from build123d import *

# Parameters (mm, degrees)
SKETCH1_W           = 70.5
SKETCH1_H           = 60
SKETCH1_R           = 2.95
BOSS_EXTRUDE1_DEPTH = 10
SKETCH3_R           = 4.5
CUT_EXTRUDE1_DEPTH  = 5
SKETCH4_W           = 10
SKETCH4_H           = 60
BOSS_EXTRUDE3_DEPTH = 31
CUT_EXTRUDE2_REACH  = 103.248
SKETCH5_R           = 12.25
SKETCH5_R_2         = 2.25
SKETCH6_W           = 60
SKETCH6_H           = 31
SKETCH6_R           = 8
BOSS_EXTRUDE4_DEPTH = 5
SKETCH7_W           = 70.5
SKETCH7_H           = 60
BOSS_EXTRUDE5_DEPTH = 5
SKETCH8_W           = 60
SKETCH8_H           = 100
SKETCH8_R           = 2.25
SKETCH8_R_2         = 20.5
BOSS_EXTRUDE6_DEPTH = 10
CUT_EXTRUDE3_REACH  = 174.876
SKETCH10_W          = 50
SKETCH10_H          = 96
SKETCH10_R          = 2.5
BOSS_EXTRUDE7_DEPTH = 10
CHAMFER1_SIZE       = 50
SKETCH11_W          = 60.5
SKETCH11_H          = 50
BOSS_EXTRUDE8_DEPTH = 10
CUT_EXTRUDE4_REACH  = 194.552
SKETCH12_R          = 4.25
CUT_EXTRUDE6_REACH  = 190.59
SKETCH14_R          = 4.25


with BuildPart() as part:
    # Sketch1 → Boss-Extrude1 (new body)
    with BuildSketch(Plane(origin=(0, 0, 0), x_dir=(1, 0, 0), z_dir=(0, 1, 0))):
        with Locations((35.25, 30)):
            Rectangle(SKETCH1_W, SKETCH1_H)
        with Locations(Location((53.25, 46, 0), (0, 0, 270))):
            Circle(SKETCH1_R, mode=Mode.SUBTRACT)
        with Locations(Location((53.25, 14, 0), (0, 0, 270))):
            Circle(SKETCH1_R, mode=Mode.SUBTRACT)
        with Locations(Location((17.25, 46, 0), (0, 0, 270))):
            Circle(SKETCH1_R, mode=Mode.SUBTRACT)
        with Locations(Location((17.25, 14, 0), (0, 0, 270))):
            Circle(SKETCH1_R, mode=Mode.SUBTRACT)
    extrude(amount=BOSS_EXTRUDE1_DEPTH)

    # Sketch3 → Cut-Extrude1 (cut)
    with BuildSketch(Plane(origin=(0, 10, 0), x_dir=(1, 0, 0), z_dir=(0, 1, 0))):
        with Locations(Location((53.25, 46, 0), (0, 0, 270))):
            Circle(SKETCH3_R)
        with Locations(Location((53.25, 14, 0), (0, 0, 270))):
            Circle(SKETCH3_R)
        with Locations(Location((17.25, 46, 0), (0, 0, 270))):
            Circle(SKETCH3_R)
        with Locations(Location((17.25, 14, 0), (0, 0, 270))):
            Circle(SKETCH3_R)
    extrude(amount=-CUT_EXTRUDE1_DEPTH, mode=Mode.SUBTRACT)

    # Sketch4 → Boss-Extrude3 (add)
    with BuildSketch(Plane(origin=(0, 10, 0), x_dir=(1, 0, 0), z_dir=(0, 1, 0))):
        with Locations((5, 30)):
            Rectangle(SKETCH4_W, SKETCH4_H)
    extrude(amount=BOSS_EXTRUDE3_DEPTH)

    # Sketch5 → Cut-Extrude2 (cut, up to next)
    with BuildSketch(Plane.ZY, mode=Mode.PRIVATE) as cut_extrude2_sk1:
        with Locations((-30, 25)):
            Circle(SKETCH5_R)
    cut_extrude2_tool1 = extrude(cut_extrude2_sk1.sketch, amount=-CUT_EXTRUDE2_REACH, mode=Mode.PRIVATE) & part.part
    # Sketch5 → Cut-Extrude2 (cut, up to next)
    with BuildSketch(Plane.ZY, mode=Mode.PRIVATE) as cut_extrude2_sk2:
        with Locations((-14, 25)):
            Circle(SKETCH5_R_2)
    cut_extrude2_tool2 = extrude(cut_extrude2_sk2.sketch, amount=-CUT_EXTRUDE2_REACH, mode=Mode.PRIVATE) & part.part
    # Sketch5 → Cut-Extrude2 (cut, up to next)
    with BuildSketch(Plane.ZY, mode=Mode.PRIVATE) as cut_extrude2_sk3:
        with Locations((-18.686291501, 36.313708499)):
            Circle(SKETCH5_R_2)
    cut_extrude2_tool3 = extrude(cut_extrude2_sk3.sketch, amount=-CUT_EXTRUDE2_REACH, mode=Mode.PRIVATE) & part.part
    # Sketch5 → Cut-Extrude2 (cut, up to next)
    with BuildSketch(Plane.ZY, mode=Mode.PRIVATE) as cut_extrude2_sk4:
        with Locations((-18.686291501, 13.686291501)):
            Circle(SKETCH5_R_2)
    cut_extrude2_tool4 = extrude(cut_extrude2_sk4.sketch, amount=-CUT_EXTRUDE2_REACH, mode=Mode.PRIVATE) & part.part
    # Sketch5 → Cut-Extrude2 (cut, up to next)
    with BuildSketch(Plane.ZY, mode=Mode.PRIVATE) as cut_extrude2_sk5:
        with Locations((-41.313708499, 36.313708499)):
            Circle(SKETCH5_R_2)
    cut_extrude2_tool5 = extrude(cut_extrude2_sk5.sketch, amount=-CUT_EXTRUDE2_REACH, mode=Mode.PRIVATE) & part.part
    # Sketch5 → Cut-Extrude2 (cut, up to next)
    with BuildSketch(Plane.ZY, mode=Mode.PRIVATE) as cut_extrude2_sk6:
        with Locations((-46, 25)):
            Circle(SKETCH5_R_2)
    cut_extrude2_tool6 = extrude(cut_extrude2_sk6.sketch, amount=-CUT_EXTRUDE2_REACH, mode=Mode.PRIVATE) & part.part
    # Sketch5 → Cut-Extrude2 (cut, up to next)
    with BuildSketch(Plane.ZY, mode=Mode.PRIVATE) as cut_extrude2_sk7:
        with Locations((-41.313708499, 13.686291501)):
            Circle(SKETCH5_R_2)
    cut_extrude2_tool7 = extrude(cut_extrude2_sk7.sketch, amount=-CUT_EXTRUDE2_REACH, mode=Mode.PRIVATE) & part.part
    add(cut_extrude2_tool1.solids().sort_by_distance((0, 25, -30))[0], mode=Mode.SUBTRACT)
    add(cut_extrude2_tool2.solids().sort_by_distance((0, 25, -14))[0], mode=Mode.SUBTRACT)
    add(cut_extrude2_tool3.solids().sort_by_distance((0, 36.313708, -18.686292))[0], mode=Mode.SUBTRACT)
    add(cut_extrude2_tool4.solids().sort_by_distance((0, 13.686292, -18.686292))[0], mode=Mode.SUBTRACT)
    add(cut_extrude2_tool5.solids().sort_by_distance((0, 36.313708, -41.313708))[0], mode=Mode.SUBTRACT)
    add(cut_extrude2_tool6.solids().sort_by_distance((0, 25, -46))[0], mode=Mode.SUBTRACT)
    add(cut_extrude2_tool7.solids().sort_by_distance((0, 13.686292, -41.313708))[0], mode=Mode.SUBTRACT)

    # Sketch6 → Boss-Extrude4 (add)
    with BuildSketch(Plane(origin=(70.5, 0, 0), x_dir=(0, 0, -1), z_dir=(1, 0, 0))):
        with Locations((30, 25.5)):
            Rectangle(SKETCH6_W, SKETCH6_H)
        with Locations((30, 25)):
            Circle(SKETCH6_R, mode=Mode.SUBTRACT)
    extrude(amount=-BOSS_EXTRUDE4_DEPTH)

    # Sketch7 → Boss-Extrude5 (add)
    with BuildSketch(Plane(origin=(0, 41, 0), x_dir=(1, 0, 0), z_dir=(0, 1, 0))):
        with Locations((35.25, 30)):
            Rectangle(SKETCH7_W, SKETCH7_H)
    extrude(amount=BOSS_EXTRUDE5_DEPTH)

    # Sketch8 → Boss-Extrude6 (add)
    with BuildSketch(Plane.ZY):
        with Locations((-30, 96)):
            Rectangle(SKETCH8_W, SKETCH8_H)
        with Locations((-53.57, 72.43)):
            Circle(SKETCH8_R, mode=Mode.SUBTRACT)
        with Locations((-6.43, 72.43)):
            Circle(SKETCH8_R, mode=Mode.SUBTRACT)
        with Locations((-6.43, 119.57)):
            Circle(SKETCH8_R, mode=Mode.SUBTRACT)
        with Locations((-53.57, 119.57)):
            Circle(SKETCH8_R, mode=Mode.SUBTRACT)
        with Locations((-30, 96)):
            Circle(SKETCH8_R_2, mode=Mode.SUBTRACT)
    extrude(amount=-BOSS_EXTRUDE6_DEPTH)

    # Sketch9 → Cut-Extrude3 (cut, up to next)
    with BuildSketch(Plane.XY, mode=Mode.PRIVATE) as cut_extrude3_sk1:
        Polygon((10, 41), (65.5, 41), (65.5, 10), (70.5, 10), (70.5, 46), (10, 46), align=None)
    cut_extrude3_tool1 = extrude(cut_extrude3_sk1.sketch, amount=-CUT_EXTRUDE3_REACH, mode=Mode.PRIVATE) & part.part
    add(cut_extrude3_tool1.solids().sort_by_distance((37.75, 41.704006, 0))[0], mode=Mode.SUBTRACT)

    # Sketch10 → Boss-Extrude7 (add)
    with BuildSketch(Plane.ZY):
        with Locations((-85, 48)):
            Rectangle(SKETCH10_W, SKETCH10_H)
        with Locations((-65.555555556, 90.444444444)):
            Circle(SKETCH10_R, mode=Mode.SUBTRACT)
        with Locations((-104.444444444, 51.555555556)):
            Circle(SKETCH10_R, mode=Mode.SUBTRACT)
        with Locations((-98.888888889, 57.111111111)):
            Circle(SKETCH10_R, mode=Mode.SUBTRACT)
        with Locations((-93.333333333, 62.666666667)):
            Circle(SKETCH10_R, mode=Mode.SUBTRACT)
        with Locations((-87.777777778, 68.222222222)):
            Circle(SKETCH10_R, mode=Mode.SUBTRACT)
        with Locations((-87.777777778, 73.777777778)):
            Circle(SKETCH10_R, mode=Mode.SUBTRACT)
        with Locations((-98.888888889, 84.888888889)):
            Circle(SKETCH10_R, mode=Mode.SUBTRACT)
        with Locations((-104.444444444, 90.444444444)):
            Circle(SKETCH10_R, mode=Mode.SUBTRACT)
        with Locations((-93.333333333, 79.333333333)):
            Circle(SKETCH10_R, mode=Mode.SUBTRACT)
        with Locations((-82.222222222, 68.222222222)):
            Circle(SKETCH10_R, mode=Mode.SUBTRACT)
        with Locations((-82.222222222, 73.777777778)):
            Circle(SKETCH10_R, mode=Mode.SUBTRACT)
        with Locations((-76.666666667, 62.666666667)):
            Circle(SKETCH10_R, mode=Mode.SUBTRACT)
        with Locations((-65.555555556, 51.555555556)):
            Circle(SKETCH10_R, mode=Mode.SUBTRACT)
        with Locations((-71.111111111, 57.111111111)):
            Circle(SKETCH10_R, mode=Mode.SUBTRACT)
        with Locations((-76.666666667, 79.333333333)):
            Circle(SKETCH10_R, mode=Mode.SUBTRACT)
        with Locations((-71.111111111, 84.888888889)):
            Circle(SKETCH10_R, mode=Mode.SUBTRACT)
    extrude(amount=-BOSS_EXTRUDE7_DEPTH)

    # Chamfer1
    chamfer1_edges = [part.edges().sort_by_distance(p)[0] for p in [
        (5, 96, -60),
    ]]
    chamfer(chamfer1_edges, length=CHAMFER1_SIZE - 0.0001)  # a hair under: the kernel refuses the full size

    # Sketch11 → Boss-Extrude8 (add)
    with BuildSketch(Plane(origin=(0, 10, 0), x_dir=(1, 0, 0), z_dir=(0, 1, 0))):
        with Locations((40.25, 85)):
            Rectangle(SKETCH11_W, SKETCH11_H)
    extrude(amount=-BOSS_EXTRUDE8_DEPTH)

    # Sketch12 → Cut-Extrude4 (cut, up to next)
    with BuildSketch(Plane(origin=(10, 0, 0), x_dir=(0, 0, -1), z_dir=(1, 0, 0)), mode=Mode.PRIVATE) as cut_extrude4_sk1:
        with Locations((85, 32.225)):
            Circle(SKETCH12_R)
    cut_extrude4_tool1 = extrude(cut_extrude4_sk1.sketch, amount=-CUT_EXTRUDE4_REACH, mode=Mode.PRIVATE) & part.part
    add(cut_extrude4_tool1.solids().sort_by_distance((10, 32.225, -85))[0], mode=Mode.SUBTRACT)

    # Sketch14 → Cut-Extrude6 (cut, up to next)
    with BuildSketch(Plane(origin=(0, 10, 0), x_dir=(1, 0, 0), z_dir=(0, 1, 0)), mode=Mode.PRIVATE) as cut_extrude6_sk1:
        with Locations(Location((32.225, 85, 0), (0, 0, 270))):
            Circle(SKETCH14_R)
    cut_extrude6_tool1 = extrude(cut_extrude6_sk1.sketch, amount=-CUT_EXTRUDE6_REACH, mode=Mode.PRIVATE) & part.part
    add(cut_extrude6_tool1.solids().sort_by_distance((32.225, 10, -85))[0], mode=Mode.SUBTRACT)

    # Mirror1: part across plane


with BuildPart() as part_1:
    add(part.part)
    add(part.part.mirror(Plane.XY.offset(-30)))


solid = part_1.part
Geometry check sheet. Reference: the model listing, model coordinates, mm. A direction names the side the tool comes from. Round coordinates to 2 decimals unless told otherwise and drop trailing zeros. Loops run counter-clockwise (first coordinate to the right, second up) from the corner with the lowest first, then second, coordinate; pieces in that order, holes last. Notation, with made-up numbers: (12, 6) -> (40, 6) arc R7 cw to (40, 19) -> close; hole circle Ø7 at (-13, -19.75). An arc over 180 degrees is marked (long way). Answer as a JSON object with one key per item and string values. Group by question number.
Item 1: Cross-section at D-D, the plane y = 105.5. Record the cut outline in (x, z), plus the area to 3 significant figures.
Item 2: Release check for a two-part mould opening along X. For faces 1 (the face through (0, 58, -29)), 2 (the face through (40, 10, -29)), 3 (the face through (18.602, 7.535, -41.708)) record: pulls with the +X half, pulls with the -X half, needs draft (parallel to the pull), parting line crosses it, or undercut.
Item 3: Set-up check for faces 4 (the face through (52, 5, -43)), 5 (the face through (4.93, 82.448, -71.653)): record each of +Z, -Z, +X, -X, +Y, -Y from which the full face is reachable in a straight line by a thin tool's end or side.
Item 4: Depth check by flat-ended pin: pin 1 Ø8 at (x, z) = (19.5, 33.5) entering from +Y; pin 2 Ø6 at (y, z) = (51.56, -65.56) entering from +X. Enter the tip coordinate at first touch or a pass-through.
Item 5: Cross-section at A-A, the plane z = -30. Record the cut outline in (x, y).
Item 6: Cross-section at B-B, the plane y = 25. Record the cut outline in (x, z), plus the area to 4 significant figures.
Item 7: Thickness scan on line 1 along X through (y, z) = (1.4, -14); line 2 along Y through (x, z) = (3, -6); line 3 along X through (y, z) = (7.7, -14). Record the ranges inside material, lowest first.
Item 8: Cross-section at C-C, the plane x = 17.25. Record the cut outline in (y, z).
Determined:
{
 "1": {"outline": "(0, -100.5) -> (10, -100.5) -> (10, -48.17) -> (0, -48.17) -> close; (0, -11.83) -> (10, -11.83) -> (10, 40.5) -> (0, 40.5) -> close", "area": "1,050 mm²"},
 "2": {"face 1": "pulls with the -X half", "face 2": "needs draft", "face 3": "undercut"},
 "3": {"face 4": "+Y", "face 5": "+X, -X"},
 "4": {"pin 1": "stops at y = 10", "pin 2": "stops at x = 10"},
 "5": {"outline": "(0, 0) -> (70.5, 0) -> (70.5, 10) -> (10, 10) -> (10, 12.75) -> (0, 12.75) -> close; (0, 37.25) -> (10, 37.25) -> (10, 75.5) -> (0, 75.5) -> close; (0, 116.5) -> (10, 116.5) -> (10, 146) -> (0, 146) -> close"},
 "6": {"outline": "(0, -110) -> (10, -110) -> (10, -48.25) -> (0, -48.25) -> close; (0, -43.75) -> (10, -43.75) -> (10, -42.25) -> (0, -42.25) -> close; (0, -17.75) -> (10, -17.75) -> (10, -16.25) -> (0, -16.25) -> close; (0, -11.75) -> (10, -11.75) -> (10, 50) -> (0, 50) -> close", "area": "1,265 mm²"},
 "7": {"line 1": "x = 0 to 14.3, 20.2 to 50.3, 56.2 to 70.5", "line 2": "y = 0 to 70.22, 74.64 to 117.36, 121.78 to 146", "line 3": "x = 0 to 12.75, 21.75 to 48.75, 57.75 to 70.5"},
 "8": {"outline": "(0, -110) -> (10, -110) -> (10, -50.5) -> (5, -50.5) -> (5, -48.95) -> (0, -48.95) -> close; (0, -43.05) -> (5, -43.05) -> (5, -41.5) -> (10, -41.5) -> (10, -18.5) -> (5, -18.5) -> (5, -16.95) -> (0, -16.95) -> close; (0, -11.05) -> (5, -11.05) -> (5, -9.5) -> (10, -9.5) -> (10, 50) -> (0, 50) -> close"}
}
